from build123d import *

# Parameters (mm, degrees)
SKETCH1_R           = 50
BOSS_EXTRUDE1_DEPTH = 80
SKETCH2_R           = 108
SKETCH2_R_2         = 50
SKETCH2_R_3         = 8
BOSS_EXTRUDE3_DEPTH = 46
BOSS_EXTRUDE4_START = 5
SKETCH3_R           = 50
BOSS_EXTRUDE4_DEPTH = 5
CHAMFER1_SIZE       = 2
CUT_EXTRUDE1_START  = -21
SKETCH6_R           = 100
SKETCH6_R_2         = 50
CUT_EXTRUDE1_DEPTH  = 21


with BuildPart() as part:
    # Sketch1 → Boss-Extrude1 (new body)
    with BuildSketch(Plane.XY):
        Circle(SKETCH1_R)
        with BuildLine():
            Line((-8, 28.4), (8, 28.4))
            Line((8, 28.4), (8, 23.685438565))
            ThreePointArc((8, 23.685438565), (0, -25), (-8, 23.685438565))
            Line((-8, 23.685438565), (-8, 28.4))
        make_face(mode=Mode.SUBTRACT)
    extrude(amount=BOSS_EXTRUDE1_DEPTH)

    # Sketch2 → Boss-Extrude3 (add)
    with BuildSketch(Plane(origin=(0, 0, 0), x_dir=(-1, 0, 0), z_dir=(0, 0, -1))):
        Circle(SKETCH2_R)
        Circle(SKETCH2_R_2, mode=Mode.SUBTRACT)
        with Locations((0, 75)):
            Circle(SKETCH2_R_3, mode=Mode.SUBTRACT)
        with Locations((75, 0)):
            Circle(SKETCH2_R_3, mode=Mode.SUBTRACT)
        with Locations((0, -75)):
            Circle(SKETCH2_R_3, mode=Mode.SUBTRACT)
        with Locations((-75, 0)):
            Circle(SKETCH2_R_3, mode=Mode.SUBTRACT)
    extrude(amount=-BOSS_EXTRUDE3_DEPTH)

    # Sketch3 → Boss-Extrude4 (add)
    with BuildSketch(Plane(origin=(0, 0, 0), x_dir=(-1, 0, 0), z_dir=(0, 0, -1)).offset(BOSS_EXTRUDE4_START)):
        Circle(SKETCH3_R)
        with BuildLine():
            Line((-8, 23.685438565), (-8, 28.4))
            Line((-8, 28.4), (8, 28.4))
            Line((8, 28.4), (8, 23.685438565))
            ThreePointArc((8, 23.685438565), (0, -25), (-8, 23.685438565))
        make_face(mode=Mode.SUBTRACT)
    extrude(amount=-BOSS_EXTRUDE4_DEPTH)

    # Chamfer1
    chamfer1_edges = [part.edges().sort_by_distance(p)[0] for p in [
        (50, 0, -5),
    ]]
    chamfer(chamfer1_edges, length=CHAMFER1_SIZE)

    # Sketch6 → Cut-Extrude1 (cut)
    with BuildSketch(Plane.XY.offset(46).offset(CUT_EXTRUDE1_START)):
        Circle(SKETCH6_R)
        Circle(SKETCH6_R_2, mode=Mode.SUBTRACT)
    extrude(amount=CUT_EXTRUDE1_DEPTH, mode=Mode.SUBTRACT)


solid = part.part
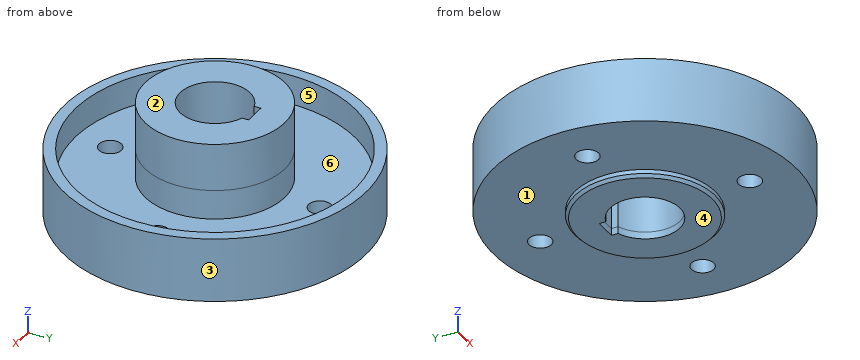
The listing builds one solid part. Answer for the finished solid, in the listing's coordinates (mm). Face numbers are marked on the shaded views. A direction names the side the tool comes from. Coordinates: 2 decimals unless noted, no trailing zeros. Write each loop counter-clockwise with the first axis right and the second up, starting at its lowest first coordinate (ties: lowest second). Pieces come first, ordered by that corner, then holes. Notation, with made-up numbers: (56, 87.5) -> (108, 87.5) arc R27 cw to (108, 111.5) -> close; hole circle Ø4 at (-19.75, -2). An arc over 180 degrees is marked (long way). One line per question, with ' | ' between items.
1. Section D-D (z = 50.5) is taken. Determine the outline of the cut face in (x, y).
Verdict:
outline: circle Ø100 at (0, 0); hole (-8, 23.69) arc R25 ccw (long way) to (8, 23.69) -> (8, 28.4) -> (-8, 28.4) -> close
2. Section B-B (y = 0) is taken. State how many separate pieces and enclosed holes the cut face has, and give its area (3 significant figures).
Verdict:
separate pieces: 4 | enclosed holes: 0 | area: 6,680 mm^2
3. Section A-A (z = 14) is taken. Determine the outline of the cut face in (x, y), and give its area (3 significant figures).
Verdict:
outline: circle Ø216 at (0, 0); hole circle Ø16 at (-75, 0); hole circle Ø16 at (0, -75); hole (-8, 23.69) arc R25 ccw (long way) to (8, 23.69) -> (8, 28.4) -> (-8, 28.4) -> close; hole circle Ø16 at (0, 75); hole circle Ø16 at (75, 0) | area: 33,800 mm^2
4. Straight lines are drawn through the part: line 1 (Y direction, x = 0, z = 11.5); line 2 (X direction, y = 0, z = 47); line 3 (Y direction, x = 0, z = -2). For each, find the intervals that lie inside material, in ascending order.
Verdict:
line 1: y = -108 to -83, -67 to -25, 28.4 to 67, 83 to 108 | line 2: x = -50 to -25, 25 to 50 | line 3: y = -50 to -25, 28.4 to 50
5. Given pin 1 Ø21 at (x, y) = (0, 75) entering from +Z; pin 2 Ø8 at (y, z) = (6.5, 29.5) entering from -X; pin 3 Ø13 at (x, y) = (-75, 0) entering from +Z; pin 4 Ø1 at (x, z) = (-56, 32) entering from -Y, each flat-ended and moving along its own axis, determine where each tip first touches the part or whether it passes through.
Verdict:
pin 1: stops at z = 25 | pin 2: stops at x = -107.97 | pin 3: passes through | pin 4: stops at y = -92.65
6. Section C-C (x = -92) is taken. Determine the outline of the cut face in (y, z), and give its area (3 significant figures).
Verdict:
outline: (-56.57, 0) -> (56.57, 0) -> (56.57, 46) -> (39.19, 46) -> (39.19, 25) -> (-39.19, 25) -> (-39.19, 46) -> (-56.57, 46) -> close | area: 3,560 mm^2
7. For a pull along Y with two mould halves and no side action, classify the marked faces 3, 4, 5 and 6 as released by +Y, released by -Y, zero draft, split by the parting line, or undercut.
Verdict:
face 3: split by the parting line | face 4: zero draft | face 5: undercut | face 6: undercut
8. Which of the six approach directions +Z, -Z, +X, -X, +Y, -Y give full straight-line access (tool end or side, diameter ignored) to the marked faces 1 and 2?
Verdict:
face 1: -Z | face 2: +Z, +X, -X, +Y, -Y
